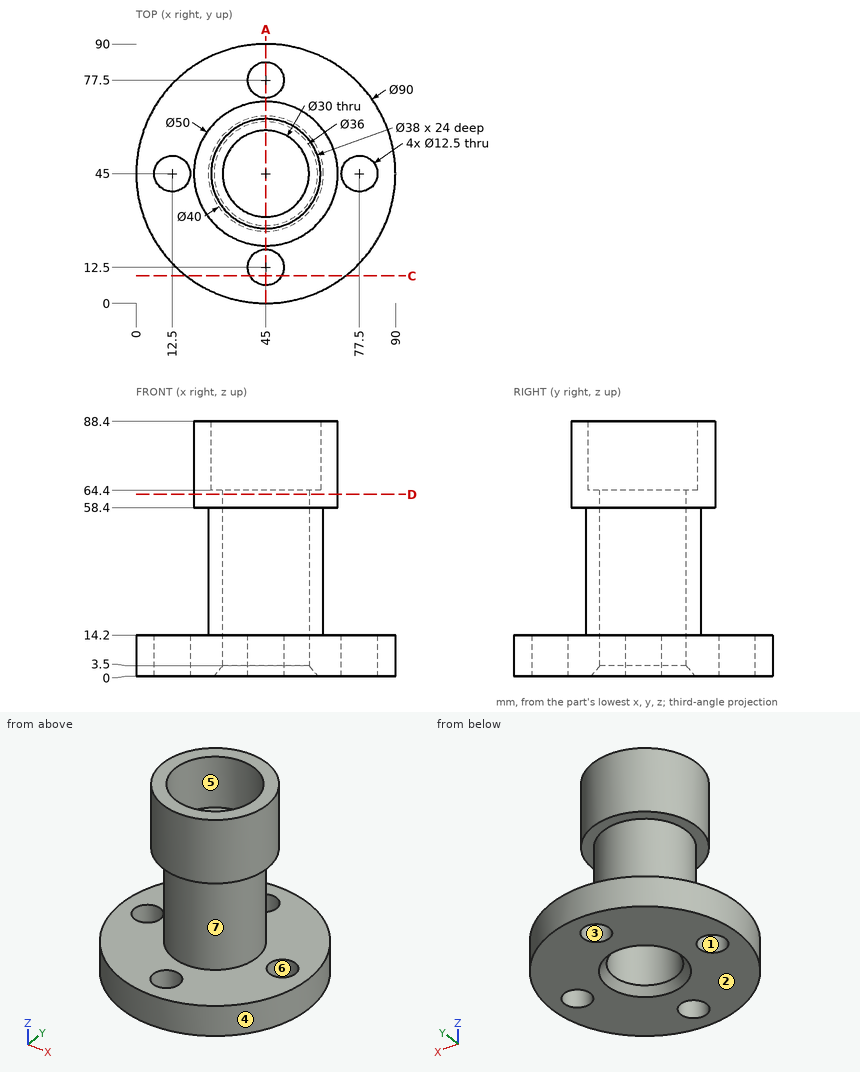
Can you work these out from the drawing? Everything is in mm from the part's minimum corner. A direction names the side the tool comes from. Round coordinates to 2 decimals unless told otherwise and drop trailing zeros. Loops run counter-clockwise (first coordinate to the right, second up) from the corner with the lowest first, then second, coordinate; pieces in that order, holes last. Notation, with made-up numbers: M 25.25,-11.75 L 69.25,-11.75 A20 ccw 69.25,15.25 Z; hole C 21,81.5 d1. An arc over 180 degrees is marked long. Answer in a Markdown table with one row per item.
1. Thinking about a two-plate mould opening in Y: for the marked faces 1, 2, 3 and 4, which applies, pulls with the +Y half, pulls with the -Y half, needs draft (parallel to the pull), parting line crosses it, or undercut?
Established:
| item | result |
|---|---|
| face 1 | undercut |
| face 2 | needs draft |
| face 3 | undercut |
| face 4 | parting line crosses it |
2. If we section it at A-A, the plane x = 45: Give the number of separate pieces and of enclosed holes in the cut face, plus the area to 3 significant figures.
Established:
| item | result |
|---|---|
| separate pieces | 4 |
| enclosed holes | 0 |
| area | 1,340 mm² |
3. If we section it at D-D, the plane z = 63: Please give me the cut outline in (x, y).
Established:
| item | result |
|---|---|
| outline | C 45,45 d50; hole C 45,45 d30 |
4. Please list where these lines run through material, in increasing order: line 1 (Y direction, x = 45, z = 36); line 2 (Y direction, x = 40.5, z = 7.5); line 3 (Z direction, x = 19.5, y = 31.5). Write a range as from..to.
Established:
| item | result |
|---|---|
| line 1 | 25..30, 60..65 |
| line 2 | 0.23..8.16, 16.84..30.69, 59.31..73.16, 81.84..89.77 |
| line 3 | 0..14.2 |
5. On a 3-axis mill with a long thin cutter (end or side, diameter ignored), from which of +Z, -Z, +X, -X, +Y, -Y can I reach the whole of each face in a straight line? I mean the marked faces 5, 6 and 7. Say none if no direction works.
Established:
| item | result |
|---|---|
| face 5 | +Z |
| face 6 | +Z, -Z |
| face 7 | none |
6. If we section it at C-C, the plane y = 9.5: Please give me the cut outline in (x, z), plus the area to 3 significant figures.
Established:
| item | result |
|---|---|
| outline | M 17.35,0 L 39.52,0 L 39.52,14.2 L 17.35,14.2 Z; M 50.48,0 L 72.65,0 L 72.65,14.2 L 50.48,14.2 Z |
| area | 630 mm² |
7. I'm going to push flat-ended pins straight in: pin 1 Ø8 at (x, y) = (53, 15.5) entering from -Z; pin 2 Ø4 at (x, y) = (31, 48) entering from -Z; pin 3 Ø14.5 at (x, y) = (12.5, 45) entering from +Z; pin 4 Ø1 at (x, z) = (35, 31) entering from +Y. Where does each tip first touch, or does it pass through?
Established:
| item | result |
|---|---|
| pin 1 | z = 0 |
| pin 2 | z = 1.96 |
| pin 3 | z = 14.2 |
| pin 4 | y = 62.6 |
